Autodesk Inventor part; units mm, degrees
ref_plane "YZ Plane" through (0, 0, 0) normal (1, 0, 0) x (0, 1, 0)
ref_plane "XZ Plane" through (0, 0, 0) normal (0, 1, 0) x (-1, 0, 0)
ref_plane "XY Plane" through (0, 0, 0) normal (0, 0, 1) x (1, 0, 0)
sketch "Sketch1" plane through (0, 0, 0) normal (0, 0, 1) x (1, 0, 0)
  line L0 (0, 0) -> (228.6, 0)
  line L1 (228.6, 0) -> (228.6, 152.4)
  line L2 (228.6, 152.4) -> (0, 152.4)
  line L3 (0, 152.4) -> (0, 0)
  line L4 (0, 152.4) -> (50.8, 152.4)
  line L5 (50.8, 152.4) -> (50.8, 0)
  line L6 (228.6, 152.4) -> (177.8, 152.4)
  line L7 (177.8, 152.4) -> (177.8, 0)
  line L8 (50.8, 0) -> (50.8, 30.48)
  line L9 (50.8, 30.48) -> (88.9, 30.48)
  circle A0 centre (88.9, 30.48) radius 2.54
  line L10 (88.9, 30.48) -> (139.7, 30.48)
  circle A1 centre (139.7, 30.48) radius 2.54
  line L11 (139.7, 30.48) -> (139.7, 106.68)
  circle A2 centre (139.7, 106.68) radius 2.54
  line L12 (88.9, 30.48) -> (88.9, 106.68)
  circle A3 centre (88.9, 106.68) radius 2.54
  line L13 (88.9, 106.68) -> (139.7, 106.68)
  line L14 (139.7, 106.68) -> (165.1, 106.68)
  circle A4 centre (165.1, 106.68) radius 2.54
  line L15 (88.9, 106.68) -> (63.5, 106.68)
  circle A5 centre (63.5, 106.68) radius 2.54
  dimension "d0" = 228.6
  dimension "d1" = 152.4
  dimension "d2" = 50.8
  dimension "d3" = 50.8
  dimension "d4" = 30.48
  dimension "d5" = 38.1
  dimension "d6" = 5.08
  dimension "d7" = 50.8
  dimension "d8" = 5.08
  dimension "d9" = 76.2
  dimension "d10" = 5.08
  dimension "d11" = 5.08
  dimension "d12" = 25.4
  dimension "d13" = 5.08
  dimension "d14" = 25.4
  dimension "d15" = 5.08
extrude "Extrusion1" add sketch "Sketch1" along normal blind 1.5875 contours L3 L2 L5 L0 | L5 L2 L7 L0 | L7 L2 L1 L0 | L12 A3 L13 A2 L11 A1 L10 A0
fillet "Fillet1" radius 3.175 4 edges at (0, 152.4, 0.7937) (228.6, 152.4, 0.7937) (228.6, 0, 0.7937) (0, 0, 0.7937)
properties part number "Kicker poly"
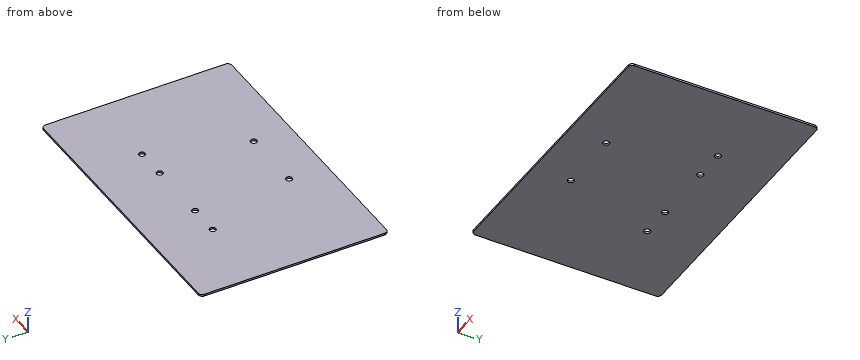
Geometry check sheet. Reference: the model listing, model coordinates, mm. Round coordinates to 2 decimals unless told otherwise and drop trailing zeros. Order: outer loops, then holes, each group sorted by start corner. A loop starts at its lowest first (then second) coordinate and runs counter-clockwise, first axis right, second up. Notation, with made-up numbers: (24.25, 58.25) - (80.25, 58.25) arc R25 cw to (80.25, 91.25) - close; hole circle Ø4 at (21, 15). An arc over 180 degrees is marked (long way). Use a Markdown table: item, result. Add a question column.
1) Gauge pin test, flat end, axial feed: P1, Ø3, axis at x = 88.9, y = 106.68, coming from the +Z side. Record the tip position at first contact, or that the pin passes through.
2) Section check C-C (y = 30.48). Record the cut outline in (x, z), then the cut area to 3 significant figures.
3) Section check A-A (y = 106.68). Record the cut outline in (x, z), then the cut area to 3 significant figures.
4) Thickness scan on line 1 along Y through (x, z) = (88.9, 1.2); line 2 along X through (y, z) = (30.48, 0.7); line 3 along Y through (x, z) = (165.1, 0.85). Record the ranges inside material, lowest first.
5) Section check B-B (x = 88.9). Record the cut outline in (y, z), then the cut area to 3 significant figures.
Established:
| question | item | result |
|---|---|---|
| 1 | P1 | through |
| 2 | outline | (0, 0) - (86.36, 0) - (86.36, 1.59) - (0, 1.59) - close; (91.44, 0) - (137.16, 0) - (137.16, 1.59) - (91.44, 1.59) - close; (142.24, 0) - (228.6, 0) - (228.6, 1.59) - (142.24, 1.59) - close |
| 2 | area | 347 mm2 |
| 3 | outline | (0, 0) - (60.96, 0) - (60.96, 1.59) - (0, 1.59) - close; (66.04, 0) - (86.36, 0) - (86.36, 1.59) - (66.04, 1.59) - close; (91.44, 0) - (137.16, 0) - (137.16, 1.59) - (91.44, 1.59) - close; (142.24, 0) - (162.56, 0) - (162.56, 1.59) - (142.24, 1.59) - close; (167.64, 0) - (228.6, 0) - (228.6, 1.59) - (167.64, 1.59) - close |
| 3 | area | 331 mm2 |
| 4 | line 1 | 0 to 27.94, 33.02 to 104.14, 109.22 to 152.4 |
| 4 | line 2 | 0 to 86.36, 91.44 to 137.16, 142.24 to 228.6 |
| 4 | line 3 | 0 to 104.14, 109.22 to 152.4 |
| 5 | outline | (0, 0) - (27.94, 0) - (27.94, 1.59) - (0, 1.59) - close; (33.02, 0) - (104.14, 0) - (104.14, 1.59) - (33.02, 1.59) - close; (109.22, 0) - (152.4, 0) - (152.4, 1.59) - (109.22, 1.59) - close |
| 5 | area | 226 mm2 |
